Here's how the part is built. I have some questions about the finished solid (model axes, mm). Face numbers are marked on the shaded views. A direction names the side the tool comes from. Coordinates: 2 decimals unless noted, no trailing zeros. Order: outer loops, then holes, each group sorted by start corner. A loop starts at its lowest first (then second) coordinate and runs counter-clockwise, first axis right, second up. Notation, with made-up numbers: (61.5, -24.5) - (81.5, -24.5) arc R22 cw to (81.5, -18.5) - close; hole circle Ø9 at (-17, 17.25). An arc over 180 degrees is marked (long way). Use CSV: the item, a comma, the result in double quotes. Start each with the question number.
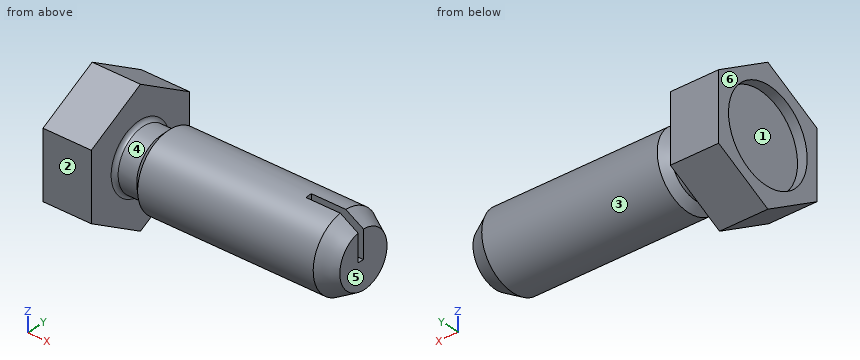
from build123d import *

# Parameters (mm, degrees)
EXTRUDE1_DEPTH           = 1.3
SKETCH11_W               = 1.4
SKETCH11_H               = 0.166666667
POINT_CUT_EXTRUDE8_DEPTH = 2.743597813
SKETCH16_R               = 1.208
CUT_EXTRUDE1_DEPTH       = 0.26


with BuildPart() as part:
    # Sketch1 → base-Revolve (revolve)
    with BuildSketch(Plane.XY):
        with BuildLine():
            Line((6, 1), (6, 0))
            Line((6, 0), (0, 0))
            Line((0, 0), (-1.04, 0))
            Line((-1.04, 0), (-1.3, 0))
            Line((-1.3, 0), (-1.3, 1.51))
            Line((-1.3, 1.51), (0, 1.51))
            Line((0, 1.51), (0, 0.9))
            ThreePointArc((0, 0.9), (0.029289322, 0.829289322), (0.1, 0.8))
            Line((0.1, 0.8), (0.6, 0.8))
            Line((0.6, 0.8), (0.8, 1))
            Line((0.8, 1), (6, 1))
        make_face()
    revolve(axis=Axis((0, 0, 0), (1, 0, 0)))

    # Sketch15 → Extrude1 (add)
    with BuildSketch(Plane.ZY.offset(1.3)):
        Polygon((-0.871798906, 1.51), (-1.743597813, 0), (-0.871798906, -1.51), (0.871798906, -1.51), (1.743597813, 0), (0.871798906, 1.51), align=None)
    extrude(amount=-EXTRUDE1_DEPTH)

    # Sketch8 → point_Cut-Revolve1 (revolve, cut)
    with BuildSketch(Plane.XY):
        Polygon((6, 0), (6.508, 0), (6.508, 1.508), (5.523686028, 1.508), (5.523686028, 1), (6, 0.725), align=None)
    revolve(axis=Axis((0, 0, 0), (1, 0, 0)), mode=Mode.SUBTRACT)

    # Sketch11 → point_Cut-Extrude8 (cut, through all)
    with BuildSketch(Plane.XY):
        with Locations((5.3, -0.083333334)):
            Rectangle(SKETCH11_W, SKETCH11_H)
    extrude(amount=POINT_CUT_EXTRUDE8_DEPTH, mode=Mode.SUBTRACT)

    # Sketch16 → Cut-Extrude1 (cut)
    with BuildSketch(Plane.ZY.offset(1.3)):
        Circle(SKETCH16_R)
    extrude(amount=-CUT_EXTRUDE1_DEPTH, mode=Mode.SUBTRACT)


solid = part.part
Item 1: Suppose I cut it at A-A on x = 4.25. Write out the boundary of the cut face in (y, z), then the cut area to 3 significant figures.
Item 2: Suppose I cut it at C-C on z = 1.5. Write out the boundary of the cut face in (x, y), then the cut area to 3 significant figures.
Item 3: For pin 1 Ø1 at (x, z) = (5, 0) entering from +Y; pin 2 Ø1.1 at (x, z) = (5, 0.5) entering from -Y; pin 3 Ø1.5 at (x, y) = (2.5, 0.5) entering from -Z, each with a flat end and sliding along its axis, tell me the tip position at first contact or that it passes through.
Item 4: We'd pull the mould along X, two halves only. Please class the marked faces 4, 5 and 6: released by +X, released by -X, zero draft, split by the parting line, or undercut.
Item 5: For the marked faces 1, 2 and 3, which set-ups out of +Z, -Z, +X, -X, +Y, -Y let a thin tool reach every point of the face, with its end or its side?
Item 6: Suppose I cut it at B-B on y = 1.1. Write out the boundary of the cut face in (x, z).
Item 7: Please list where these lines run through material, in increasing order: line 1 along Y through (x, z) = (-1.2, 0); line 2 along X through (y, z) = (0.8, -0.8); line 3 along Y through (x, z) = (3, -0.6). Write a range as from..to.
Here are the results:
1,outline,"circle Ø2 at (0, 0)"
1,area,"3.14 mm^2"
2,outline,"(-1.3, -0.42) - (0, -0.42) - (0, 0.42) - (-1.3, 0.42) - close"
2,area,"1.10 mm^2"
3,pin 1,"y = 1"
3,pin 2,"y = -1"
3,pin 3,"z = -1"
4,face 4,"undercut"
4,face 5,"released by +X"
4,face 6,"released by -X"
5,face 1,"-X"
5,face 2,"+Z, -Z, +X, -X, -Y"
5,face 3,"+X"
6,outline,"(-1.3, -1.11) - (0, -1.11) - (0, 1.11) - (-1.3, 1.11) - (-1.3, 0.5) - (-1.04, 0.5) - (-1.04, -0.5) - (-1.3, -0.5) - close"
7,line 1,"-1.51..-1.21, 1.21..1.51"
7,line 2,"-1.04..0"
7,line 3,"-0.8..0.8"
